Could you check a few things on this model? Use its own coordinates, in mm. A direction names the side the tool comes from. Round coordinates to 2 decimals unless told otherwise and drop trailing zeros. Loops run counter-clockwise (first coordinate to the right, second up) from the corner with the lowest first, then second, coordinate; pieces in that order, holes last. Notation, with made-up numbers: (33, 52.5) - (70, 52.5) arc R32 cw to (70, 83.5) - close; hole circle Ø1 at (24, 46). An arc over 180 degrees is marked (long way). Put each result on its own line as item: value. Start each with the question number.
Autodesk Inventor part; units mm, degrees
ref_plane "YZ Plane" through (0, 0, 0) normal (1, 0, 0) x (0, 1, 0)
ref_plane "XZ Plane" through (0, 0, 0) normal (0, 1, 0) x (-1, 0, 0)
ref_plane "XY Plane" through (0, 0, 0) normal (0, 0, 1) x (1, 0, 0)
sketch "Sketch1" plane through (0, 0, 0) normal (0, 0, 1) x (1, 0, 0)
  circle A0 centre (0, 0) radius 0.75
  circle A1 centre (0, 0) radius 1.75
  dimension "d0" = 1.5
  dimension "d1" = 3.5
extrude "Extrusion1" add sketch "Sketch1" along normal mid plane 10 contours A0
extrude "Extrusion2" add sketch "Sketch1" along normal blind 1
fillet "Fillet1" radius 1 1 edges at (-1.75, 0, 1)
properties part number "X-Ray Tube Pins" material "Aluminum 6061"
Item 1: Will these pins go through, and if not, where does the flat tip stop? P1, Ø1, axis at y = 0, z = -2, coming from the +X side; P2, Ø1, axis at x = 1, z = -3.5, coming from the -Y side.
Item 2: On a 3-axis mill with a long thin cutter (end or side, diameter ignored), from which of +Z, -Z, +X, -X, +Y, -Y can I reach the whole of each face in a straight line? I mean faces 1 (the face through (-0.75, -0.03, 2.97)), 2 (the face through (-0.75, 0.03, -2.46)), 3 (the face through (0, 0, 5)). Say none if no direction works.
Item 3: Suppose I cut it at A-A, the plane z = -0.25. List the corners of the cut face in (x, y) for me, then the cut area to 3 significant figures.
Item 4: I need wall thicknesses on line 1 (Z direction, x = -0.05, y = -0.8); line 2 (X direction, y = -0.05, z = 1.25); line 3 (Y direction, x = 0.6, z = 4.5). Which ranges of each line are inside material? Lowest first, please. Write a range as from..to.
Numbers:
1. P1: x = 0.75
1. P2: y = -0.56
2. face 1: +Z
2. face 2: -Z
2. face 3: +Z, +X, -X, +Y, -Y
3. outline: circle Ø1.5 at (0, 0)
3. area: 1.77 mm^2
4. line 1: 0..1
4. line 2: -0.75..0.75
4. line 3: -0.45..0.45
